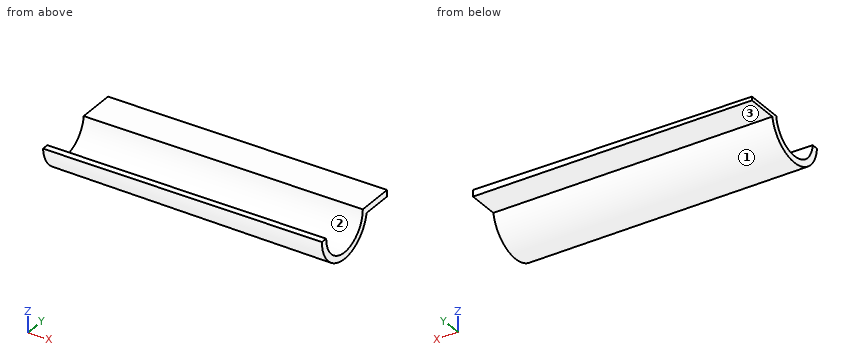
```python
from build123d import *

# Parameters (mm, degrees)
F1_DEPTH = 149.999954
F3_DEPTH = 78.74


with BuildPart() as f1:
    # F0 (on Right) → F1 (new body)
    with BuildSketch(Plane.YZ):
        with BuildLine():
            ThreePointArc((-86.749771, 0), (-101.735771, -14.986), (-116.721771, 0))
            Line((-116.721771, 0), (-120.221764, 0))
            ThreePointArc((-120.221764, 0), (-103.493734, -18.402215), (-83.584132, -3.499993))
            Line((-83.584132, -3.499993), (-66.937771, -3.499993))
            Line((-66.937771, -3.499993), (-66.937771, 0))
            Line((-66.937771, 0), (-86.749771, 0))
        make_face()
    extrude(amount=F1_DEPTH)

    # F2 (on face) → F3 (cut)
    with BuildSketch(Plane(origin=(0, -66.937771, 0), x_dir=(-1, 0, 0), z_dir=(0, 1, 0))):
        Polygon((0, 0), (-149.999954, 0), (0, -1.531896), align=None)
    extrude(amount=-F3_DEPTH, mode=Mode.SUBTRACT)


solid = f1.part
```
CAD build for the part. Positions are in the model's coordinates, mm. Face numbers are marked on the shaded views. Coordinates: 2 decimals unless noted, no trailing zeros. Order: outer loops, then holes, each group sorted by start corner. A loop starts at its lowest first (then second) coordinate and runs counter-clockwise, first axis right, second up. Notation, with made-up numbers: (46, 57) -> (81, 57) arc R16 ccw to (81, 62) -> close; hole circle Ø1 at (-38.5, 11.5). An arc over 180 degrees is marked (long way). Use one line per item in the form item = value. Start each with the question number.
1) Band-saw the part on A-A on z = -7.25. Give the cut face in (x, y), then the cut area to 3 significant figures.
2) Band-saw the part on C-C on y = -72. Give the cut face in (x, z), then the cut area to 3 significant figures.
3) Pull direction Y, two halves, no side cores. Call the marked faces 1, 2 and 3: +Y half, -Y half, draft (parallel to the pull), parting line (faces both ways), or undercut.
4) Band-saw the part on D-D on x = 13. Give the cut face in (y, z), then the cut area to 3 significant figures.
5) Band-saw the part on B-B on x = 28.5. Give the cut face in (y, z), then the cut area to 3 significant figures.
6) Drill centre lines: L1, parallel to Z at x = 139.5, y = -101; L2, parallel to Y at x = 144, z = -1.75; L3, parallel to Y at x = 47, z = -10.25. Where is each one in solid material? Low to high. Write a range as [from, to].
7) Drop flat-ended pins along their axis: pin 1 (1 mm diameter, centred on y = -89.5, z = -3.5, fed in from -X); pin 2 (13.5 mm diameter, centred on x = 112, y = -74, fed in from -Z); pin 3 (8 mm diameter, centred on x = 133.5, z = -8, fed in from -Y); pin 4 (1 mm diameter, centred on x = 41, y = -96, fed in from +Z). Give the stop position or say it passes through.
Entries:
q1.outline = (0, -118.74) -> (150, -118.74) -> (150, -114.85) -> (0, -114.85) -> close; (0, -88.62) -> (150, -88.62) -> (150, -84.73) -> (0, -84.73) -> close
q1.area = 1,170 mm2
q2.outline = (0, -3.5) -> (150, -3.5) -> (150, 0) -> (0, -1.53) -> close
q2.area = 410 mm2
q3.face_1 = parting line
q3.face_2 = undercut
q3.face_3 = draft
q4.outline = (-120.17, -1.4) arc R18.49 ccw to (-83.58, -3.5) -> (-66.94, -3.5) -> (-66.94, -1.4) -> (-86.82, -1.4) arc R14.99 cw to (-116.66, -1.4) -> close
q4.area = 209 mm2
q5.outline = (-120.18, -1.24) arc R18.49 ccw to (-83.58, -3.5) -> (-66.94, -3.5) -> (-66.94, -1.24) -> (-86.8, -1.24) arc R14.99 cw to (-116.67, -1.24) -> close
q5.area = 213 mm2
q6.L1 = [-18.47, -14.97]
q6.L2 = [-120.14, -116.62], [-86.85, -66.94]
q6.L3 = [-117.12, -112.67], [-90.8, -86.35]
q7.pin_1 = through
q7.pin_2 = -3.5
q7.pin_3 = -119.78
q7.pin_4 = -13.63
